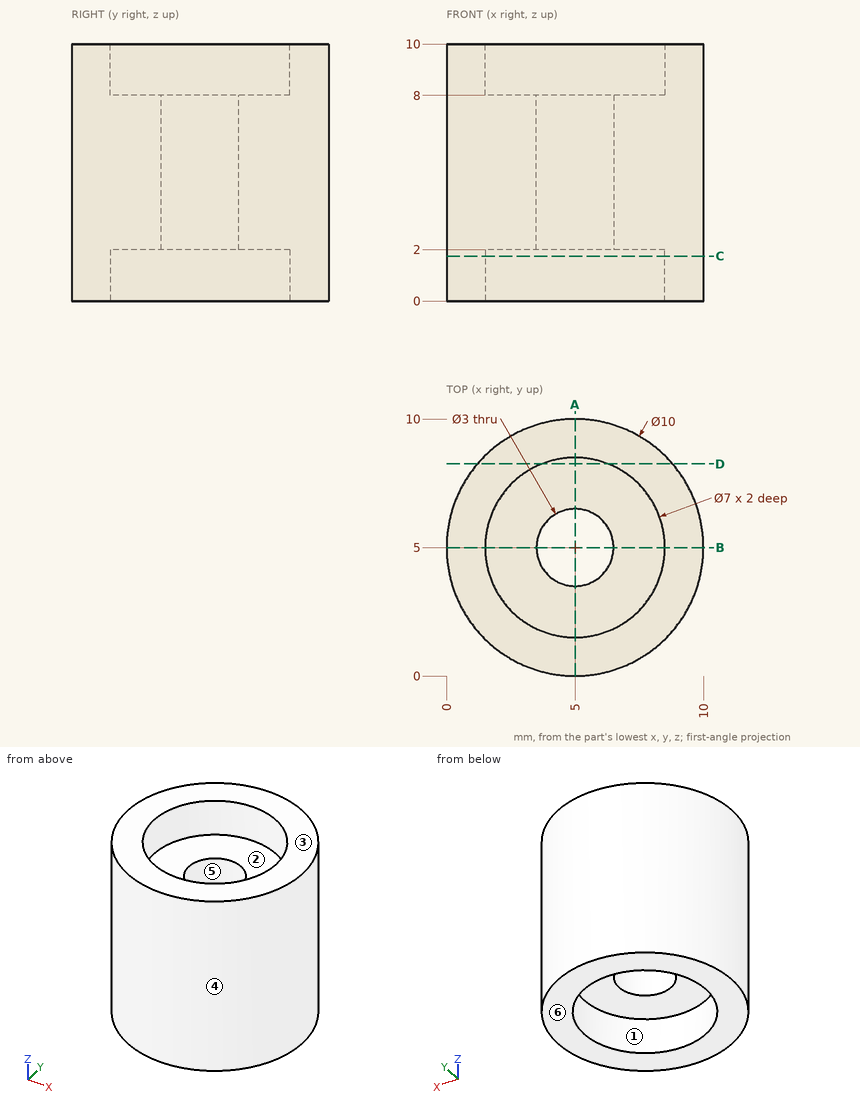
Answer from the drawing. Dimensions are ordinates in mm from the lowest x, y and z of the part. A direction names the side the tool comes from. Round coordinates to 2 decimals unless told otherwise and drop trailing zeros. Loops run counter-clockwise (first coordinate to the right, second up) from the corner with the lowest first, then second, coordinate; pieces in that order, holes last.
Q1. Section D-D on y = 8.25 is taken. Write down the section's boundary in (x, z).
Q2. Each of these flat-tipped pins is pushed along its axis until it touches: pin 1 (5 mm diameter, centred on x = 6.5, z = 2, fed in from -Y); pin 2 (5 mm diameter, centred on x = 5, y = 5, fed in from -Z); pin 3 (3.5 mm diameter, centred on x = 4.5, y = 6, fed in from +Z); pin 4 (1 mm diameter, centred on y = 7, z = 8.5, fed in from +X). Where does it stop, or does it pass through?
Q3. Which of the six approach directions +Z, -Z, +X, -X, +Y, -Y give full straight-line access (tool end or side, diameter ignored) to the marked faces 1, 2 and 3?
Q4. Section A-A on x = 5 is taken. Write down the section's boundary in (y, z).
Q5. Consider probe 1 along Y at (x, z) = (5, 1); probe 2 along Z at (x, y) = (4.5, 2.5); probe 3 along X at (y, z) = (5.25, 2.75). Determine where each line is inside the solid, lowest interval first.
Q6. Determine the mould class of the marked faces 4, 5 and 6 for opening direction Y: released by +Y, released by -Y, zero draft, split by the parting line, or undercut.
Q7. Section C-C on z = 1.75 is taken. Write down the section's boundary in (x, y).
Output:
1. outline: (1.2, 0) - (3.7, 0) - (3.7, 2) - (6.3, 2) - (6.3, 0) - (8.8, 0) - (8.8, 10) - (6.3, 10) - (6.3, 8) - (3.7, 8) - (3.7, 10) - (1.2, 10) - close
2. pin 1: stops at y = 0
2. pin 2: stops at z = 2
2. pin 3: stops at z = 8
2. pin 4: stops at x = 9.77
3. face 1: -Z
3. face 2: +Z
3. face 3: +Z, +X, -X, +Y, -Y
4. outline: (0, 0) - (1.5, 0) - (1.5, 2) - (3.5, 2) - (3.5, 8) - (1.5, 8) - (1.5, 10) - (0, 10) - close; (6.5, 2) - (8.5, 2) - (8.5, 0) - (10, 0) - (10, 10) - (8.5, 10) - (8.5, 8) - (6.5, 8) - close
5. probe 1: y = 0 to 1.5, 8.5 to 10
5. probe 2: z = 2 to 8
5. probe 3: x = 0.01 to 3.52, 6.48 to 9.99
6. face 4: split by the parting line
6. face 5: undercut
6. face 6: zero draft
7. outline: circle Ø10 at (5, 5); hole circle Ø7 at (5, 5)
